Model file for the job. Use its own axes, mm. Round coordinates to 2 decimals unless told otherwise and drop trailing zeros. Order: outer loops, then holes, each group sorted by start corner. A loop starts at its lowest first (then second) coordinate and runs counter-clockwise, first axis right, second up. Notation, with made-up numbers: (77.25, 27) - (125.25, 27) arc R9 cw to (125.25, 36) - close; hole circle Ø6 at (54, 28.25). An arc over 180 degrees is marked (long way). Write item = value, one per line. Start each with the question number.
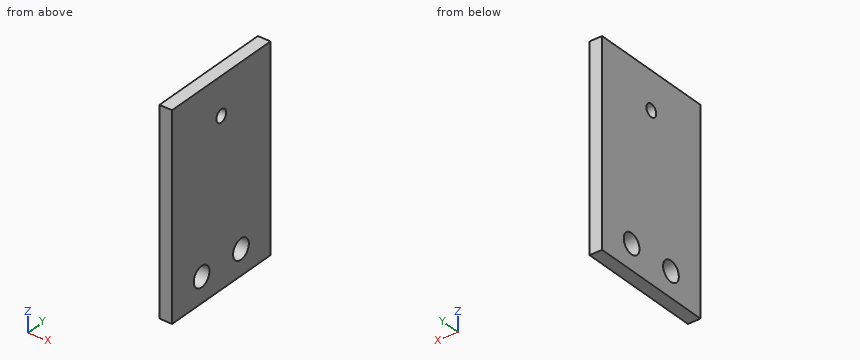
Autodesk Inventor part; units mm, degrees
ref_plane "YZ Plane" through (0, 0, 0) normal (1, 0, 0) x (0, 1, 0)
ref_plane "XZ Plane" through (0, 0, 0) normal (0, 1, 0) x (-1, 0, 0)
ref_plane "XY Plane" through (0, 0, 0) normal (0, 0, 1) x (1, 0, 0)
sketch "Skizze1" plane through (0, 0, 0) normal (1, 0, 0) x (0, 1, 0)
  line L0 (0, 0) -> (50, 0)
  line L1 (50, 0) -> (50, -80)
  line L2 (50, -80) -> (0, -80)
  line L3 (0, -80) -> (0, 0)
  dimension "d0" = 50
  dimension "d1" = 80
extrude "Extrusion1" add sketch "Skizze1" along normal blind 5
sketch "Skizze2" plane through (5, 0, 0) normal (1, 0, 0) x (0, 0, -1)
  line L0 (0, 0) -> (80, 0)
  line L1 (80, 0) -> (70, 0)
  line L2 (70, 0) -> (70, 15)
  line L3 (70, 15) -> (70, 35)
  line L4 (70, 35) -> (70, 50)
  dimension "d4" = 10
  dimension "d5" = 15
  dimension "d6" = 20
  dimension "d7" = 15
hole "Bohrung1" at (5, 35, -70) at (5, 15, -70) direction (-1, 0, 0) diameter 8 depth 8 tip angle 118
sketch "Skizze3" plane through (5, 0, 0) normal (1, 0, 0) x (0, 0, -1)
  line L0 (0, 0) -> (0, 25)
  line L1 (0, 50) -> (0, 0)
  line L2 (0, 25) -> (15, 25)
  circle A0 centre (15, 25) radius 2.5
  dimension "d15" = 25
  dimension "d16" = 15
  dimension "d17" = 5
extrude "Extrusion2" cut sketch "Skizze3" against normal blind 10
properties part number "Stuetzplatte"
Item 1: Saw through at A-A, the plane y = 25. Give the cut face in (x, z), then the cut area to 3 significant figures.
Item 2: Saw through at B-B, the plane x = 2.35. Give the cut face in (y, z).
Item 3: Saw through at C-C, the plane z = -70.5. Give the cut face in (x, y).
Item 4: Saw through at D-D, the plane y = 35. Give the cut face in (x, z).
Item 5: Probe L1, parallel to Y at x = 3.95, z = -70; L2, parallel to Z at x = 4, y = 15; L3, parallel to Y at x = 2.95, z = -73.5. List the from-to ranges inside material, lowest first.
Check sheet entries:
q1.outline = (0, -80) - (5, -80) - (5, -17.5) - (0, -17.5) - close; (0, -12.5) - (5, -12.5) - (5, 0) - (0, 0) - close
q1.area = 375 mm2
q2.outline = (0, -80) - (50, -80) - (50, 0) - (0, 0) - close; hole circle Ø8 at (15, -70); hole circle Ø5 at (25, -15); hole circle Ø8 at (35, -70)
q3.outline = (0, 0) - (5, 0) - (5, 11.03) - (0, 11.03) - close; (0, 18.97) - (5, 18.97) - (5, 31.03) - (0, 31.03) - close; (0, 38.97) - (5, 38.97) - (5, 50) - (0, 50) - close
q4.outline = (0, -80) - (5, -80) - (5, -74) - (0, -74) - close; (0, -66) - (5, -66) - (5, 0) - (0, 0) - close
q5.L1 = 0 to 11, 19 to 31, 39 to 50
q5.L2 = -80 to -74, -66 to 0
q5.L3 = 0 to 13.06, 16.94 to 33.06, 36.94 to 50
